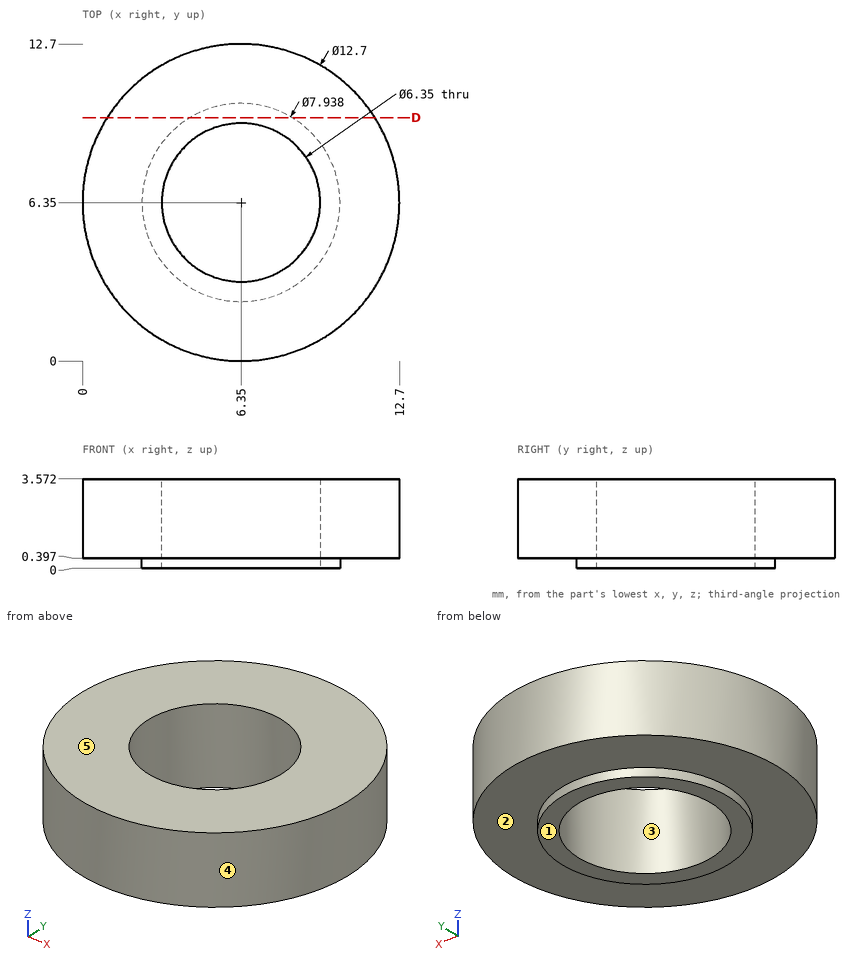
Could you check a few things on this drawing? It's one solid part, dimensions in mm from its lowest x, y, z. A direction names the side the tool comes from. Coordinates: 2 decimals unless noted, no trailing zeros. Loops run counter-clockwise (first coordinate to the right, second up) from the corner with the lowest first, then second, coordinate; pieces in that order, holes last. Notation, with made-up numbers: (52, 42.5) - (83, 42.5) arc R29 ccw to (83, 77.5) - close; hole circle Ø1 at (21, 46.25). An arc over 180 degrees is marked (long way). Answer as a JSON object with one key per item and string values. Group by question number.
Item 1: For pin 1 (2 mm diameter, centred on x = 1.5, z = 0.5, fed in from -Y); pin 2 (1 mm diameter, centred on y = 4.5, z = 2, fed in from +X) (1 decimal); pin 3 (1 mm diameter, centred on y = 5, z = 1, fed in from -X), each with a flat end and sliding along its axis, tell me the tip position at first contact or that it passes through.
Item 2: If we section it at D-D (y = 9.75): List the corners of the cut face in (x, z) for me.
Item 3: If we mould it in two halves opening along Y, with no side actions, what happens to the marked faces 3, 4 and 5? For each: released by +Y, released by -Y, zero draft, split by the parting line, or undercut.
Item 4: If I drill on L1, parallel to Y at x = 6.35, z = 0.8 (1 decimal); L2, parallel to Z at x = 4.25, y = 12.25; L3, parallel to X at y = 6.25, z = 3, over which ranges is the centre line in solid material (lowest first)? Write a range as from..to.
Item 5: On a 3-axis mill with a long thin cutter (end or side, diameter ignored), from which of +Z, -Z, +X, -X, +Y, -Y can I reach the whole of each face in a straight line? I mean the marked faces 1 and 2. Say none if no direction works.
Returned:
{
 "1": {"pin 1": "stops at y = 1.3", "pin 2": "stops at x = 12.6", "pin 3": "stops at x = 0.06"},
 "2": {"outline": "(0.99, 0.4) - (4.3, 0.4) - (4.3, 0) - (8.4, 0) - (8.4, 0.4) - (11.71, 0.4) - (11.71, 3.57) - (0.99, 3.57) - close"},
 "3": {"face 3": "undercut", "face 4": "split by the parting line", "face 5": "zero draft"},
 "4": {"L1": "y = 0..3.2, 9.5..12.7", "L2": "z = 0.4..3.57", "L3": "x = 0..3.18, 9.52..12.7"},
 "5": {"face 1": "-Z, +X, -X, +Y, -Y", "face 2": "-Z"}
}
